```python
from build123d import *

# Parameters (mm, degrees)
SKETCH1_R           = 10
BOSS_EXTRUDE2_DEPTH = 8
SKETCH3_R           = 10
SKETCH3_R_2         = 6
CUT_EXTRUDE1_DEPTH  = 5
SKETCH4_R           = 2.1
CUT_EXTRUDE2_DEPTH  = 11
SKETCH5_R           = 6
CUT_EXTRUDE3_DEPTH  = 1.5
SKETCH6_R           = 6.5
CUT_EXTRUDE4_DEPTH  = 2
SKETCH7_R           = 6
CUT_EXTRUDE5_DEPTH  = 1
SKETCH8_R           = 6
CUT_EXTRUDE6_DEPTH  = 1
SKETCH9_R           = 6.5
BOSS_EXTRUDE3_DEPTH = 2
CUT_EXTRUDE7_DEPTH  = 10


with BuildPart() as part:
    # Sketch1 → Boss-Extrude2 (new body)
    with BuildSketch(Plane(origin=(0, 0, 0), x_dir=(1, 0, 0), z_dir=(0, 1, 0))):
        Circle(SKETCH1_R)
    extrude(amount=BOSS_EXTRUDE2_DEPTH)

    # Sketch3 → Cut-Extrude1 (cut)
    with BuildSketch(Plane(origin=(0, 8, 0), x_dir=(1, 0, 0), z_dir=(0, 1, 0))):
        Circle(SKETCH3_R)
        Circle(SKETCH3_R_2, mode=Mode.SUBTRACT)
    extrude(amount=-CUT_EXTRUDE1_DEPTH, mode=Mode.SUBTRACT)

    # Sketch4 → Cut-Extrude2 (cut)
    with BuildSketch(Plane(origin=(0, 8, 0), x_dir=(1, 0, 0), z_dir=(0, 1, 0))):
        Circle(SKETCH4_R)
    extrude(amount=-CUT_EXTRUDE2_DEPTH, mode=Mode.SUBTRACT)

    # Sketch5 → Cut-Extrude3 (cut)
    with BuildSketch(Plane.XZ):
        Circle(SKETCH5_R)
    extrude(amount=-CUT_EXTRUDE3_DEPTH, mode=Mode.SUBTRACT)

    # Sketch6 → Cut-Extrude4 (cut)
    with BuildSketch(Plane.XZ):
        Circle(SKETCH6_R)
    extrude(amount=-CUT_EXTRUDE4_DEPTH, mode=Mode.SUBTRACT)

    # Sketch7 → Cut-Extrude5 (cut)
    with BuildSketch(Plane(origin=(0, 8, 0), x_dir=(1, 0, 0), z_dir=(0, 1, 0))):
        Circle(SKETCH7_R)
    extrude(amount=-CUT_EXTRUDE5_DEPTH, mode=Mode.SUBTRACT)

    # Sketch8 → Cut-Extrude6 (cut)
    with BuildSketch(Plane(origin=(0, 7, 0), x_dir=(1, 0, 0), z_dir=(0, 1, 0))):
        Circle(SKETCH8_R)
    extrude(amount=-CUT_EXTRUDE6_DEPTH, mode=Mode.SUBTRACT)

    # Sketch9 → Boss-Extrude3 (add)
    with BuildSketch(Plane.XZ.offset(-2)):
        Circle(SKETCH9_R)
        Polygon((-3.6, -2.1), (0, -4.1), (3.6, -2.1), (3.6, 2.1), (0, 4.1), (-3.6, 2.1), align=None, mode=Mode.SUBTRACT)
    extrude(amount=BOSS_EXTRUDE3_DEPTH)

    # Sketch10 → Cut-Extrude7 (cut)
    with BuildSketch(Plane(origin=(0, 0, 0), x_dir=(-1, 0, 0), z_dir=(0, -1, 0))):
        with BuildLine():
            ThreePointArc((-4.358898944, -9), (0, -10), (4.358898944, -9))
            Line((4.358898944, -9), (-4.358898944, -9))
        make_face()
        with BuildLine():
            ThreePointArc((4.358898944, 9), (0, 10), (-4.358898944, 9))
            Line((-4.358898944, 9), (4.358898944, 9))
        make_face()
    extrude(amount=-CUT_EXTRUDE7_DEPTH, mode=Mode.SUBTRACT)


solid = part.part
```
Can you work these out from the model? Positions are in its coordinate system, mm. A direction names the side the tool comes from. Coordinates: 2 decimals unless noted, no trailing zeros. Write each loop counter-clockwise with the first axis right and the second up, starting at its lowest first coordinate (ties: lowest second). Pieces come first, ordered by that corner, then holes. Notation, with made-up numbers: M -21,41 L 4,41 A13 cw 4,63 Z; hole C -4.5,26.25 d1. An arc over 180 degrees is marked long. Answer as CSV lines item,"result".
Item 1: Please list where these lines run through material, in increasing order: line 1 along Z through (x, y) = (0, 3.7); line 2 along Y through (x, z) = (8, -0.5).
Geometry results:
line 1,"z = -6 to -2.1, 2.1 to 6"
line 2,"y = 0 to 3"
Item 2: On a 3-axis mill with a long thin cutter (end or side, diameter ignored), from which of +Z, -Z, +X, -X, +Y, -Y can I reach the whole of each face in a straight line? I mean faces 5 (the flat face through (-1.8, 1, 3.1)), 6 (the flat face through (0, 1, 9)). Say none if no direction works.
Geometry results:
face 5,"-Y"
face 6,"+Z, +X, -X, +Y, -Y"
Item 3: Imagine slicing it at B-B on x = 1.5. List the corners of the cut face in (y, z) for me.
Geometry results:
outline,"M 0,-9 L 3,-9 L 3,-5.81 L 6,-5.81 L 6,-1.47 L 2,-1.47 L 2,-3.27 L 0,-3.27 Z; M 0,3.27 L 2,3.27 L 2,1.47 L 6,1.47 L 6,5.81 L 3,5.81 L 3,9 L 0,9 Z"
Item 4: Imagine slicing it at C-C on y = 4.1. List the corners of the cut face in (x, z) for me, plus the area to 3 significant figures.
Geometry results:
outline,"C 0,0 d12; hole C 0,0 d4.2"
area,"99.2 mm2"
Item 5: Imagine slicing it at D-D on z = 5.25. List the corners of the cut face in (x, y) for me.
Geometry results:
outline,"M -8.51,0 L 8.51,0 L 8.51,3 L 2.9,3 L 2.9,6 L -2.9,6 L -2.9,3 L -8.51,3 Z"
Item 6: We'd pull the mould along Z, two halves only. Please class faces 1 (the cylindrical face through (-6, 5, 0)), 2 (the flat face through (-5, 3, -4)), 3 (the flat face through (1.8, 1, 3.1)), 4 (the flat face through (-1.8, 1, -3.1)): +Z half, -Z half, draft (parallel to the pull), parting line (faces both ways), or undercut.
Geometry results:
face 1,"parting line"
face 2,"draft"
face 3,"undercut"
face 4,"undercut"
Item 7: I'm going to push flat-ended pins straight in: P1, Ø3, axis at y = 1.5, z = 4.5, coming from the +X side; P2, Ø3.5, axis at x = -1, z = -1, coming from the -Y side; P3, Ø4, axis at x = -8, z = 7, coming from the +Y side. Where does each tip first touch, or does it pass through?
Geometry results:
P1,"stops at x = 9.54"
P2,"stops at y = 2"
P3,"stops at y = 3"
Item 8: Imagine slicing it at A-A on z = 0. List the corners of the cut face in (x, y) for me.
Geometry results:
outline,"M -10,0 L -3.6,0 L -3.6,2 L -2.1,2 L -2.1,6 L -6,6 L -6,3 L -10,3 Z; M 2.1,2 L 3.6,2 L 3.6,0 L 10,0 L 10,3 L 6,3 L 6,6 L 2.1,6 Z"
